from build123d import *

# Parameters (mm, degrees)
F0_W         = 82
F0_H         = 35
F1_DEPTH     = 1
F2_W         = 72
F2_H         = 25
F3_DEPTH     = 7
F5_DEPTH     = 2
F6_R         = 2
F7_DEPTH     = 2
F8_W         = 67
F8_H         = 17
F9_DEPTH     = 0.2
F10_T1_DEPTH = 20
F10_T3_DEPTH = 70
F11_R        = 0.5
F12_DEPTH    = 2


# Not quite as in the source:
# - a fillet or chamfer that OpenCascade refuses, or shapes differently, is made with other operations: its cross-section is extruded or revolved along the edge and cut away or added


with BuildPart() as f1:
    # F0 (on Top) → F1 (new body)
    with BuildSketch(Plane.XY):
        Rectangle(F0_W, F0_H)
    extrude(amount=F1_DEPTH)

    # F2 (on face) → F3 (join)
    with BuildSketch(Plane.XY.offset(1)):
        with Locations((0, -2)):
            Rectangle(F2_W, F2_H)
    extrude(amount=F3_DEPTH)

    # F4 (on face) → F5 (join)
    with BuildSketch(Plane.XY.offset(1)):
        Polygon((36, -10.5), (41, -5.5), (41, 1.5), (36, 6.5), align=None)
    extrude(amount=F5_DEPTH)

    # F6 (on face) → F7 (cut)
    with BuildSketch(Plane.XY.offset(1)):
        with Locations((-38.5, -15)):
            Circle(F6_R)
        with Locations((38.5, -15)):
            Circle(F6_R)
        with Locations((-38.5, 15)):
            Circle(F6_R)
        with Locations((38.5, 15)):
            Circle(F6_R)
    extrude(amount=-F7_DEPTH, mode=Mode.SUBTRACT)

    # F8 (on face) → F9 (cut)
    with BuildSketch(Plane.XY.offset(8)):
        with Locations((0, -2)):
            Rectangle(F8_W, F8_H)
    extrude(amount=-F9_DEPTH, mode=Mode.SUBTRACT)

    # F10: fillet of radius 1 on 4 edges, made by hand

    # F10_s2 → F10_t1 (join)
    with BuildSketch(Plane.XZ.offset(-8)):
        with BuildLine():
            ThreePointArc((33.5, 8), (33.216227766, 7.8513167019), (32.9, 7.8))
            Line((32.9, 7.8), (33.5, 7.8))
            Line((33.5, 7.8), (33.5, 8))
        make_face()
        with BuildLine():
            ThreePointArc((-33.5, 8), (-33.216227766, 7.8513167019), (-32.9, 7.8))
            Line((-32.9, 7.8), (-33.5, 7.8))
            Line((-33.5, 7.8), (-33.5, 8))
        make_face()
    extrude(amount=F10_T1_DEPTH)

    # F10_s4 → F10_t3 (join)
    with BuildSketch(Plane.YZ.offset(-35)):
        with BuildLine():
            ThreePointArc((6.5, 8), (6.216227766, 7.8513167019), (5.9, 7.8))
            Line((5.9, 7.8), (6.5, 7.8))
            Line((6.5, 7.8), (6.5, 8))
        make_face()
        with BuildLine():
            ThreePointArc((-10.5, 8), (-10.216227766, 7.8513167019), (-9.9, 7.8))
            Line((-9.9, 7.8), (-10.5, 7.8))
            Line((-10.5, 7.8), (-10.5, 8))
        make_face()
    extrude(amount=F10_T3_DEPTH)

    # F11 (on face) → F12 (cut)
    with BuildSketch(Plane.XY.offset(1)):
        with Locations((-33.5, 15)):
            Circle(F11_R)
        with Locations((-31, 15)):
            Circle(F11_R)
        with Locations((-28.5, 15)):
            Circle(F11_R)
        with Locations((-26, 15)):
            Circle(F11_R)
        with Locations((-23.5, 15)):
            Circle(F11_R)
        with Locations((-21, 15)):
            Circle(F11_R)
        with Locations((-18.5, 15)):
            Circle(F11_R)
        with Locations((-16, 15)):
            Circle(F11_R)
        with Locations((-13.5, 15)):
            Circle(F11_R)
        with Locations((-11, 15)):
            Circle(F11_R)
        with Locations((-8.5, 15)):
            Circle(F11_R)
        with Locations((-6, 15)):
            Circle(F11_R)
        with Locations((-3.5, 15)):
            Circle(F11_R)
        with Locations((-1, 15)):
            Circle(F11_R)
        with Locations((1.5, 15)):
            Circle(F11_R)
        with Locations((4, 15)):
            Circle(F11_R)
    extrude(amount=-F12_DEPTH, mode=Mode.SUBTRACT)


solid = f1.part
Verification items for the finished model (mm, model axes). A direction names the side the tool comes from. Give positions to 0.01 mm unless a question says otherwise; leave off trailing zeros. Loops run counter-clockwise (first coordinate to the right, second up) from the corner with the lowest first, then second, coordinate; pieces in that order, holes last.
1) Sectioned sample at D-D, the plane z = 6. Enter the section's corners in (x, y).
2) Draft check along Y on faces 1 (the cylindrical face through (-39.974, -13.648, 0.507)), 2 (the flat face through (38.5, 4, 2)), 3 (the flat face through (36, -2, 5)). Enter one of: pulls with the +Y half, pulls with the -Y half, needs draft (parallel to the pull), parting line crosses it, or undercut.
3) Depth check by flat-ended pin: pin 1 Ø4 at (x, z) = (7, 4.5) entering from +Y; pin 2 Ø4.5 at (x, y) = (8, -1.5) entering from +Z; pin 3 Ø1.5 at (y, z) = (-6.5, 2) entering from +X. Enter the tip coordinate at first touch or a pass-through.
4) Sectioned sample at A-A, the plane x = 38.5. Enter the section's corners in (y, z).
5) Sectioned sample at B-B, the plane z = 2. Enter the section's corners in (x, y).
6) Set-up check for faces 4 (the flat face through (-36, -2, 4)), 5 (the flat face through (0, -2, 7.8)), 6 (the flat face through (38, -2, 3)), 7 (the flat face through (-1, -14.5, 4)): record each of +Z, -Z, +X, -X, +Y, -Y from which the full face is reachable in a straight line by a thin tool's end or side.
7) Sectioned sample at C-C, the plane x = -38.5. Enter the section's corners in (y, z).
8) Thickness scan on line 1 along Y through (x, z) = (-13.5, 0.75); line 2 along Y through (x, z) = (-38.5, 0.8); line 3 along Y through (x, z) = (27, 5.5). Record the ranges inside material, lowest first.
Answers:
1. outline: (-36, -14.5) - (36, -14.5) - (36, 10.5) - (-36, 10.5) - close
2. face 1: undercut
2. face 2: pulls with the +Y half
2. face 3: needs draft
3. pin 1: stops at y = 10.5
3. pin 2: stops at z = 7.8
3. pin 3: stops at x = 40.75
4. outline: (-17.5, 0) - (-17, 0) - (-17, 1) - (-17.5, 1) - close; (-13, 0) - (13, 0) - (13, 1) - (4, 1) - (4, 3) - (-8, 3) - (-8, 1) - (-13, 1) - close; (17, 0) - (17.5, 0) - (17.5, 1) - (17, 1) - close
5. outline: (-36, -14.5) - (36, -14.5) - (36, -10.5) - (41, -5.5) - (41, 1.5) - (36, 6.5) - (36, 10.5) - (-36, 10.5) - close
6. face 4: +Z, -X, +Y, -Y
6. face 5: +Z
6. face 6: +Z, +X, +Y, -Y
6. face 7: +Z, +X, -X, -Y
7. outline: (-17.5, 0) - (-17, 0) - (-17, 1) - (-17.5, 1) - close; (-13, 0) - (13, 0) - (13, 1) - (-13, 1) - close; (17, 0) - (17.5, 0) - (17.5, 1) - (17, 1) - close
8. line 1: y = -17.5 to 14.5, 15.5 to 17.5
8. line 2: y = -17.5 to -17, -13 to 13, 17 to 17.5
8. line 3: y = -14.5 to 10.5
